Job drawing, mm, ordinate dimensions from the low corner. One solid piece. A direction names the side the tool comes from. Coordinates: 2 decimals unless noted, no trailing zeros. Order: outer loops, then holes, each group sorted by start corner. A loop starts at its lowest first (then second) coordinate and runs counter-clockwise, first axis right, second up. Notation, with made-up numbers: (48, 37.5) - (63, 37.5) arc R31 ccw to (63, 75.5) - close; hole circle Ø8 at (-7, 0.25). An arc over 180 degrees is marked (long way). Use a Markdown table: item, result. Add a question column.
1) Saw through at C-C on x = 2.5. List the corners of the cut face in (y, z), then the cut area to 3 significant figures.
2) Wall check: L1, parallel to Y at x = 7, z = 1.75; L2, parallel to Y at x = 7, z = 13.5; L3, parallel to X at y = 7, z = 4.75 (1 decimal). Give the ranges that are in metal, low to high. Write a range as [from, to].
3) Two-plate mould, pull along X, no slides. Class the marked faces 3, 4 and 5: +X half, -X half, draft (parallel to the pull), parting line (faces both ways), or undercut.
4) Tool access for the marked faces 1 and 2: list every direction of +Z, -Z, +X, -X, +Y, -Y with a clear straight run to the whole face (end or side of a thin tool).
5) Drop flat-ended pins along their axis: P1, Ø4, axis at y = 5.5, z = 13.5, coming from the +X side; P2, Ø1.5, axis at x = 4.5, z = 10, coming from the -Y side. Give the stop position or say it passes through.
6) Saw through at A-A on x = 5.5. List the corners of the cut face in (y, z), then the cut area to 3 significant figures.
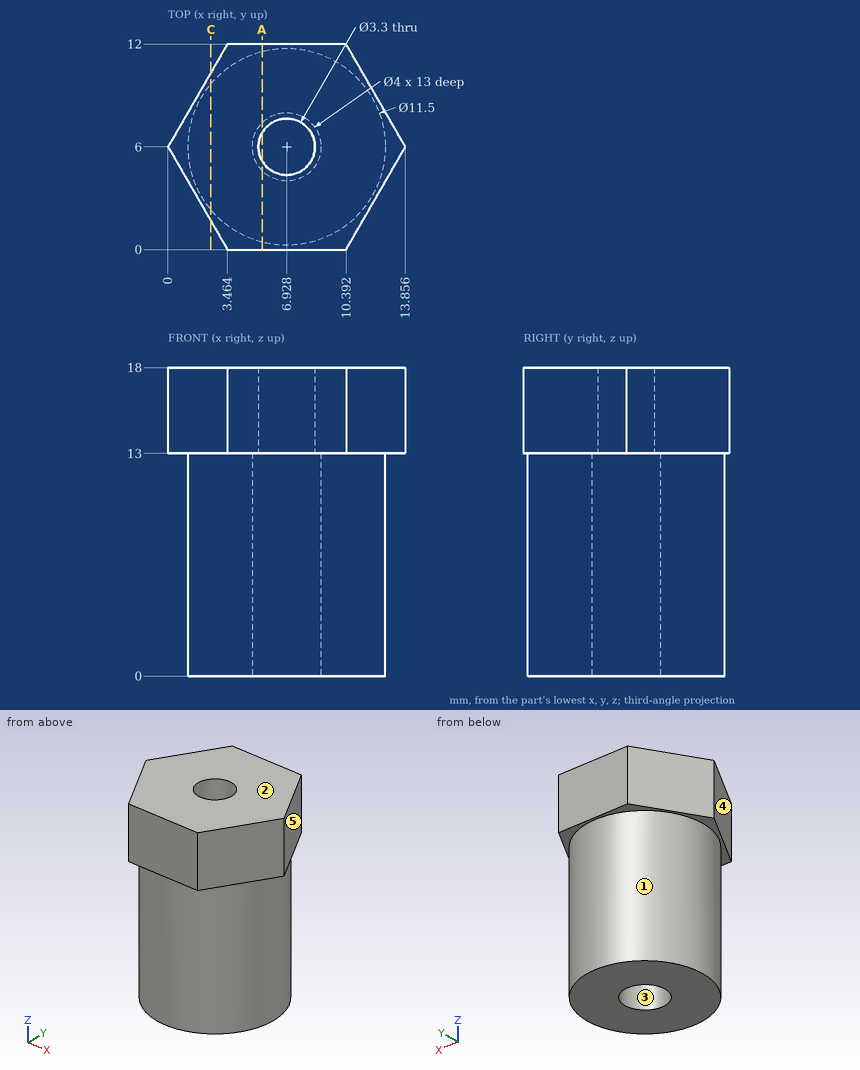
Results are:
| question | item | result |
|---|---|---|
| 1 | outline | (1.67, 13) - (2.33, 13) - (2.33, 0) - (9.67, 0) - (9.67, 13) - (10.33, 13) - (10.33, 18) - (1.67, 18) - close |
| 1 | area | 139 mm2 |
| 2 | L1 | [0.25, 4], [8, 11.75] |
| 2 | L2 | [0, 4.35], [7.65, 12] |
| 2 | L3 | [1.3, 5.2], [8.7, 12.6] |
| 3 | face 3 | undercut |
| 3 | face 4 | -X half |
| 3 | face 5 | +X half |
| 4 | face 1 | -Z |
| 4 | face 2 | +Z, +X, -X, +Y, -Y |
| 5 | P1 | x = 13.86 |
| 5 | P2 | y = 0.5 |
| 6 | outline | (0, 13) - (0.43, 13) - (0.43, 0) - (4.6, 0) - (4.6, 13) - (5.17, 13) - (5.17, 18) - (0, 18) - close; (6.83, 13) - (7.4, 13) - (7.4, 0) - (11.57, 0) - (11.57, 13) - (12, 13) - (12, 18) - (6.83, 18) - close |
| 6 | area | 160 mm2 |
